Geometry: final body of the model. Coordinates: model frame, mm. A direction names the side the tool comes from. Give positions to 0.01 mm unless a question says otherwise; leave off trailing zeros. Write each loop counter-clockwise with the first axis right and the second up, starting at its lowest first coordinate (ties: lowest second). Pieces come first, ordered by that corner, then holes. Notation, with made-up numbers: (25, 3.5) - (33, 3.5) arc R30 cw to (33, 32.5) - close; hole circle Ø5 at (-12, 63). An arc over 180 degrees is marked (long way). Use CSV: the item, a comma, the result in double quotes. Start each with the question number.
(1) Reachability of faces 1 (the flat face through (22, -10, 0)), 2 (the flat face through (18, -13, 0)), 3 (the flat face through (18, 1, -17)) from +Z, -Z, +X, -X, +Y, -Y: full face, straight path, thin tool, end or side. Return the list, or none.
(2) Section B-B on z = 0. Output: boundary loops of the cut face in (x, y).
(3) First-contact query: pin 1 Ø2 at (y, z) = (0.5, 15.5) entering from +X; pin 2 Ø1.5 at (y, z) = (-17.5, -9) entering from -X; pin 3 Ø12 at (x, z) = (-15.5, 13) entering from -Y; pin 4 Ø10 at (x, y) = (-9, -6.5) entering from -Z. Flat tips, straight axial feed; report the tip coordinate or a pass-through.
(4) Section D-D on z = -19. Output: boundary loops of the cut face in (x, y).
(5) Line query: probe 1 along Z at (x, y) = (-14, 1.25); probe 2 along X at (y, z) = (1.55, 0); probe 3 along Y at (x, z) = (-3, -7). Output: solid intervals per line, ascending. Write a range as [from, to].
(6) Section C-C on y = -19.75. Output: boundary loops of the cut face in (x, z).
(7) Section A-A on x = -14. Output: boundary loops of the cut face in (y, z), and give its area (3 significant figures).
(8) Draft query along Z for faces 4 (the cylindrical face through (-8.46, 1.01, 2.3)), 5 (the flat face through (-2, 1, 21.5)), 6 (the cylindrical face through (20.028, -16.503, -0.253)), 7 (the flat face through (18, 1, 17)). Return one class per face: released by +Z, released by -Z, zero draft, split by the parting line, or undercut.
Autodesk Inventor part; units mm, degrees
ref_plane "YZ Plane" through (0, 0, 0) normal (1, 0, 0) x (0, 1, 0)
ref_plane "XZ Plane" through (0, 0, 0) normal (0, 1, 0) x (-1, 0, 0)
ref_plane "XY Plane" through (0, 0, 0) normal (0, 0, 1) x (1, 0, 0)
sketch "Sketch1" plane through (0, 0, 0) normal (0, 1, 0) x (-1, 0, 0)
  line L0 (-22, 21.5) -> (22, 21.5)
  line L1 (22, 21.5) -> (22, -21.5)
  line L2 (22, -21.5) -> (-22, -21.5)
  line L3 (-22, -21.5) -> (-22, 21.5)
  line L4 (-22, 21.5) -> (22, -21.5) construction
  line L5 (22, 21.5) -> (-22, -21.5) construction
  line L6 (-22, 21.5) -> (-18, 21.5)
  line L7 (-18, 21.5) -> (-18, 12.5)
  line L8 (-18, 12.5) -> (-22, 12.5)
  line L9 (-22, 12.5) -> (-22, 21.5)
  line L10 (-22, -21.5) -> (-18, -21.5)
  line L11 (-18, -21.5) -> (-18, -12.5)
  line L12 (-18, -12.5) -> (-22, -12.5)
  line L13 (-22, -12.5) -> (-22, -21.5)
  point P0 (0, 0)
  point P1 (-22, 12.5)
  dimension "d0" = 44
  dimension "d1" = 43
  dimension "d7" = 4
  dimension "d8" = 9
  dimension "d9" = 4
  dimension "d10" = 9
extrude "Extrusion1" add sketch "Sketch1" along normal blind 2 contours L0 L1 L2 L11 L12 L3 L8 L7
sketch "Sketch3" plane through (0, 2, 0) normal (0, 1, 0) x (1, 0, 0)
  line L0 (18, -12.5) -> (22, -12.5)
  line L1 (22, -12.5) -> (22, 12.5)
  line L2 (18, -12.5) -> (22, -12.5)
  line L3 (22, -12.5) -> (22, 12.5)
  line L4 (22, 12.5) -> (18, 12.5)
  line L5 (18, 12.5) -> (18, -12.5)
  point P0 (0, 0)
extrude "Extrusion3" add sketch "Sketch3" against normal blind 30
sketch "Sketch4" plane through (22, 2, 12.5) normal (1, 0, 0) x (0, 0, -1)
  line L0 (0, -30) -> (25, -30)
  circle A0 centre (12.5, -30) radius 11.5
  point P0 (12.5, -2)
  dimension "d13" = 23
extrude "Extrusion4" cut sketch "Sketch4" against normal blind 4
sketch "Sketch5" plane through (0, 2, 0) normal (0, 1, 0) x (1, 0, 0)
  line L0 (-22, 21.5) -> (-22, -21.5)
  line L1 (-22, 0) -> (-14, 0)
  line L2 (-22, 0) -> (-14, 0) construction
  circle A0 centre (-14, 0) radius 6
  point P0 (0, 0)
  dimension "d16" = 8
  dimension "d17" = 0
  dimension "d18" = 12
extrude "Extrusion5" cut sketch "Sketch5" against normal through all
fillet "Fillet1" radius 4 1 edges at (18, 0, 0)
properties part number "Stepper_Closing_2"
Check values:
1,face 1,"+Z, -Z, +X, +Y, -Y"
1,face 2,"+Z, -Z, -X, -Y"
1,face 3,"-Z, +X, +Y, -Y"
2,outline,"(-22, 0) - (-20, 0) - (-20, 2) - (-22, 2) - close; (-8, 0) - (14, 0) arc R4 cw to (18, -4) - (18, -16.5) - (22, -16.5) - (22, 2) - (-8, 2) - close"
3,pin 1,"stops at x = 18"
3,pin 2,"stops at x = 18"
3,pin 3,"stops at y = 0"
3,pin 4,"passes through"
4,outline,"(-22, 0) - (18, 0) - (18, 2) - (-22, 2) - close"
5,probe 1,"z = [-21.5, -6], [6, 21.5]"
5,probe 2,"x = [-22, -20], [-8, 22]"
5,probe 3,"y = [0, 2]"
6,outline,"(18, -12.5) - (22, -12.5) - (22, -8.01) - (18, -8.01) - close; (18, 8.01) - (22, 8.01) - (22, 12.5) - (18, 12.5) - close"
7,outline,"(0, -21.5) - (2, -21.5) - (2, -6) - (0, -6) - close; (0, 6) - (2, 6) - (2, 21.5) - (0, 21.5) - close"
7,area,"62.0 mm²"
8,face 4,"undercut"
8,face 5,"released by +Z"
8,face 6,"undercut"
8,face 7,"zero draft"
